from build123d import *

# Parameters (mm, degrees)
SKETCH1_R           = 0.15
BOSS_EXTRUDE1_DEPTH = 0.6


with BuildPart() as part:
    # Sketch1 → Boss-Extrude1 (new body)
    with BuildSketch(Plane.XY):
        Polygon((148.35, 52.1), (148.35, 51.1), (147.85, 51.1), (147.85, 48.1), (148.35, 48.1), (148.35, 47.1), (146.55, 47.1), (146.05, 47.1), (140.55, 47.1), (140.05, 47.1), (139.15, 47.1), (139.15, 48.3), (139.15, 49.3), (139.15, 52.1), align=None)
        with Locations((147.87, 47.6)):
            Circle(SKETCH1_R, mode=Mode.SUBTRACT)
        with Locations((147.87, 51.6)):
            Circle(SKETCH1_R, mode=Mode.SUBTRACT)
    extrude(amount=BOSS_EXTRUDE1_DEPTH)


solid = part.part
For this review, take the finished solid that the model builds, in its own axes (mm). Give positions to 0.01 mm unless a question says otherwise; leave off trailing zeros. Loops run counter-clockwise (first coordinate to the right, second up) from the corner with the lowest first, then second, coordinate; pieces in that order, holes last. Notation, with made-up numbers: M 31,9 L 85,9 A34 ccw 85,48 Z; hole C 20.5,70.25 d7. An arc over 180 degrees is marked long. Put each result on its own line as item: value. Start each with the question number.
(1) Wall thickness on L1, parallel to X at y = 47.6, z = 0.15; L2, parallel to X at y = 50.15, z = 0.4: over which ranges is each line inside the solid? List them lowest first.
(2) Add section D-D, the plane y = 50.65. Write out the cut boundary in (x, z), then the cut area to 3 significant figures.
(3) Add section A-A, the plane z = 0.2. Write out the cut boundary in (x, y).
(4) Add section B-B, the plane x = 148.25. Write out the cut boundary in (y, z), then the cut area to 3 significant figures.
(5) Add section C-C, the plane y = 47.6. Write out the cut boundary in (x, z).
Result:
1. L1: x = 139.15 to 147.72, 148.02 to 148.35
1. L2: x = 139.15 to 147.85
2. outline: M 139.15,0 L 147.85,0 L 147.85,0.6 L 139.15,0.6 Z
2. area: 5.22 mm^2
3. outline: M 139.15,47.1 L 148.35,47.1 L 148.35,48.1 L 147.85,48.1 L 147.85,51.1 L 148.35,51.1 L 148.35,52.1 L 139.15,52.1 Z; hole C 147.87,47.6 d0.3; hole C 147.87,51.6 d0.3
4. outline: M 47.1,0 L 48.1,0 L 48.1,0.6 L 47.1,0.6 Z; M 51.1,0 L 52.1,0 L 52.1,0.6 L 51.1,0.6 Z
4. area: 1.20 mm^2
5. outline: M 139.15,0 L 147.72,0 L 147.72,0.6 L 139.15,0.6 Z; M 148.02,0 L 148.35,0 L 148.35,0.6 L 148.02,0.6 Z
